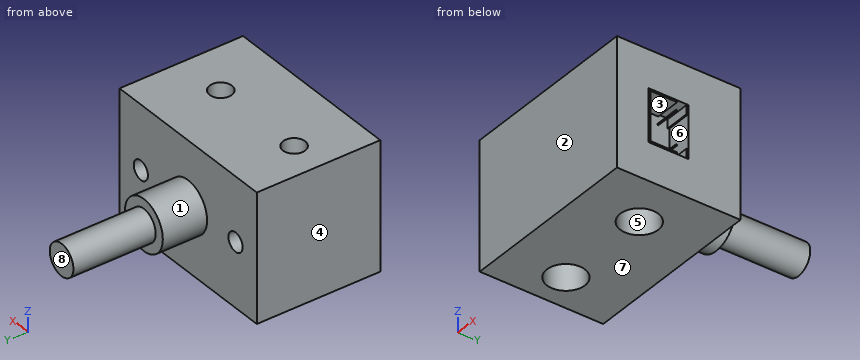
```python
from build123d import *

# Parameters (mm, degrees)
SKETCH1_W                              = 29
SKETCH1_H                              = 19.5
SKETCH1_R                              = 1.75
FRONTPROFILEBOSS_EXTRUDE1_DEPTH        = 20.2
SKETCH2_R                              = 1.5
TOPMOUNTINGHOLESCUT_EXTRUDE1_DEPTH     = 4
SKETCH3_R                              = 4
CONNINGTOWERBOSS_EXTRUDE2_DEPTH        = 7
SKETCH4_R                              = 2.5
PLUNGERBOSS_EXTRUDE3_DEPTH             = 13
SKETCH5_R                              = 3
BACKMOUNTINGHOLESBORCUT_EXTRUDE2_DEPTH = 6
SKETCH6_W                              = 8.3
SKETCH6_H                              = 6.3
XHTERMINALCUT_EXTRUDE14_DEPTH          = 4
SKETCH7_W                              = 1.4
SKETCH7_H                              = 0.2
SKETCH7_W_2                            = 0.15
SKETCH7_H_2                            = 0.15
XHTERMINALBOSS_EXTRUDE4_DEPTH          = 4


with BuildPart() as part:
    # Sketch1 → FrontProfileBoss-Extrude1 (new body)
    with BuildSketch(Plane.XY):
        with Locations((14.5, 9.75)):
            Rectangle(SKETCH1_W, SKETCH1_H)
        with Locations((5.5, 9.5)):
            Circle(SKETCH1_R, mode=Mode.SUBTRACT)
        with Locations((21, 9.5)):
            Circle(SKETCH1_R, mode=Mode.SUBTRACT)
    extrude(amount=FRONTPROFILEBOSS_EXTRUDE1_DEPTH)

    # Sketch2 → TopMountingHolesCut-Extrude1 (cut)
    with BuildSketch(Plane(origin=(0, 19.5, 0), x_dir=(1, 0, 0), z_dir=(0, 1, 0))):
        with Locations(Location((4.5, -10.1, 0), (0, 0, 270))):
            Circle(SKETCH2_R)
        with Locations(Location((24.5, -10.1, 0), (0, 0, 270))):
            Circle(SKETCH2_R)
    extrude(amount=-TOPMOUNTINGHOLESCUT_EXTRUDE1_DEPTH, mode=Mode.SUBTRACT)

    # Sketch3 → ConningTowerBoss-Extrude2 (add)
    with BuildSketch(Plane(origin=(0, 19.5, 0), x_dir=(1, 0, 0), z_dir=(0, 1, 0))):
        with Locations(Location((14.5, -10.1, 0), (0, 0, 90))):
            Circle(SKETCH3_R)
    extrude(amount=CONNINGTOWERBOSS_EXTRUDE2_DEPTH)

    # Sketch4 → PlungerBoss-Extrude3 (add)
    with BuildSketch(Plane(origin=(0, 26.5, 0), x_dir=(1, 0, 0), z_dir=(0, 1, 0))):
        with Locations(Location((14.5, -10.1, 0), (0, 0, 90))):
            Circle(SKETCH4_R)
    extrude(amount=PLUNGERBOSS_EXTRUDE3_DEPTH)

    # Sketch5 → BackMountingHolesBorCut-Extrude2 (cut)
    with BuildSketch(Plane(origin=(0, 0, 0), x_dir=(-1, 0, 0), z_dir=(0, 0, -1))):
        with Locations((-21, 9.5)):
            Circle(SKETCH5_R)
        with Locations((-5.5, 9.5)):
            Circle(SKETCH5_R)
    extrude(amount=-BACKMOUNTINGHOLESBORCUT_EXTRUDE2_DEPTH, mode=Mode.SUBTRACT)

    # Sketch6 → XHTerminalCut-Extrude14 (cut)
    with BuildSketch(Plane(origin=(29, 0, 0), x_dir=(0, 0, -1), z_dir=(1, 0, 0))):
        with Locations((-10.1, 8.15)):
            Rectangle(SKETCH6_W, SKETCH6_H)
    extrude(amount=-XHTERMINALCUT_EXTRUDE14_DEPTH, mode=Mode.SUBTRACT)

    # Sketch7 → XHTerminalBoss-Extrude4 (add)
    with BuildSketch(Plane(origin=(25, 0, 0), x_dir=(0, 0, -1), z_dir=(1, 0, 0))):
        Polygon((-14.15, 9.5), (-14.15, 5.1), (-6.05, 5.1), (-6.05, 9.5), (-6.25, 9.5), (-6.25, 5.3), (-13.95, 5.3), (-13.95, 9.5), align=None)
        with Locations((-13.45, 11.1)):
            Rectangle(SKETCH7_W, SKETCH7_H)
        with Locations((-6.75, 11.1)):
            Rectangle(SKETCH7_W, SKETCH7_H)
        with Locations((-12.675, 9.425)):
            Rectangle(SKETCH7_W_2, SKETCH7_H_2)
        with Locations((-7.375, 9.425)):
            Rectangle(SKETCH7_W_2, SKETCH7_H_2)
    extrude(amount=XHTERMINALBOSS_EXTRUDE4_DEPTH)


solid = part.part
```
For this review, take the finished solid that the model builds, in its own axes (mm). Face numbers are marked on the shaded views. A direction names the side the tool comes from. Give positions to 0.01 mm unless a question says otherwise; leave off trailing zeros. Write each loop counter-clockwise with the first axis right and the second up, starting at its lowest first coordinate (ties: lowest second). Pieces come first, ordered by that corner, then holes.
Item 1: Take a section at C-C (x = 14.5). Give the boundary of the cut face in (y, z).
Item 2: Take a section at D-D (y = 25). Give the boundary of the cut face in (x, z).
Item 3: Take a section at A-A (x = 4.5). Give the boundary of the cut face in (y, z).
Item 4: Insertion check: P1, Ø6, axis at x = 13.5, z = 5, coming from the +Y side; P2, Ø2, axis at x = 17.5, z = 6, coming from the +Y side; P3, Ø4, axis at x = 16, y = 25.5, coming from the -Z side; P4, Ø4, axis at x = 21, y = 9.5, coming from the -Z side. Each pin has a flat end and moves straight along its axis. Give the tip position at first contact, or say it passes through.
Item 5: Machinability: for the marked faces 1, 2, 3, 4 and 5, which of the approach directions +Z, -Z, +X, -X, +Y, -Y give a long, thin tool a straight path to every point of the face, cutting with its end or side? Answer none if there is none.
Item 6: The part is to be moulded in two halves that separate along Z. For the marked faces 6, 7 and 8, say which applies: +Z half, -Z half, draft (parallel to the pull), parting line (faces both ways), or undercut.
Item 7: Wall thickness on probe 1 along X at (y, z) = (9.5, 11); probe 2 along Y at (x, z) = (5.5, 13); probe 3 along Y at (x, z) = (5.5, 3.6): over which ranges is each line inside the solid? List them lowest first.
Item 8: Take a section at B-B (z = 18.25). Give the boundary of the cut face in (x, y).
Established:
1. outline: (0, 0) - (19.5, 0) - (19.5, 6.1) - (26.5, 6.1) - (26.5, 7.6) - (39.5, 7.6) - (39.5, 12.6) - (26.5, 12.6) - (26.5, 14.1) - (19.5, 14.1) - (19.5, 20.2) - (0, 20.2) - close
2. outline: circle Ø8 at (14.5, 10.1)
3. outline: (0, 0) - (6.67, 0) - (6.67, 6) - (8.06, 6) - (8.06, 20.2) - (0, 20.2) - close; (10.94, 6) - (12.33, 6) - (12.33, 0) - (19.5, 0) - (19.5, 8.6) - (15.5, 8.6) - (15.5, 11.6) - (19.5, 11.6) - (19.5, 20.2) - (10.94, 20.2) - close
4. P1: stops at y = 39.5
4. P2: stops at y = 19.5
4. P3: stops at z = 6.1
4. P4: stops at z = 6
5. face 1: +Y
5. face 2: +Z, -Z, +X, -X, -Y
5. face 3: +X
5. face 4: +Z, -Z, -X, +Y, -Y
5. face 5: -Z
6. face 6: undercut
6. face 7: -Z half
6. face 8: draft
7. probe 1: x = 0 to 3.75, 7.25 to 19.25, 22.75 to 25
7. probe 2: y = 0 to 7.75, 11.25 to 19.5
7. probe 3: y = 0 to 6.5, 12.5 to 19.5
8. outline: (0, 0) - (29, 0) - (29, 19.5) - (0, 19.5) - close; hole circle Ø3.5 at (5.5, 9.5); hole circle Ø3.5 at (21, 9.5)
